from build123d import *

# Parameters (mm, degrees)
SKETCH1_W                = 100
SKETCH1_H                = 64
BOSS_EXTRUDE1_DEPTH      = 3
SKETCH2_W                = 100
SKETCH2_H                = 64
SKETCH2_W_2              = 96
SKETCH2_H_2              = 60
BOSS_EXTRUDE2_DEPTH      = 35
SKETCH6_R                = 3
SKETCH6_R_2              = 1.6
BOSS_EXTRUDE3_DEPTH      = 10
SKETCH7_R                = 1.5
CUT_EXTRUDE2_DEPTH       = 69.912988616
BOSS_EXTRUDE8_START      = -10
SKETCH10_R               = 3
SKETCH10_W               = 10
SKETCH10_H               = 10.5
SKETCH10_H_2             = 10
BOSS_EXTRUDE8_DEPTH      = 6
SKETCH11_R               = 3
CUT_EXTRUDE4_DEPTH       = 3
BOSS_EXTRUDE9_DEPTH      = 5
BOSS_EXTRUDE9_DEPTH_BACK = 37
SKETCH12_W               = 5
SKETCH12_H               = 5
SKETCH13_W               = 5.5
SKETCH13_H               = 5.5
CUT_EXTRUDE5_DEPTH       = 7
FILLET1_R                = 10


with BuildPart() as part:
    # Sketch1 → Boss-Extrude1 (new body)
    with BuildSketch(Plane(origin=(0, 0, 0), x_dir=(1, 0, 0), z_dir=(0, 1, 0))):
        Rectangle(SKETCH1_W, SKETCH1_H)
    extrude(amount=BOSS_EXTRUDE1_DEPTH)

    # Sketch2 → Boss-Extrude2 (add)
    with BuildSketch(Plane(origin=(0, 3, 0), x_dir=(1, 0, 0), z_dir=(0, 1, 0))):
        Rectangle(SKETCH2_W, SKETCH2_H)
        Rectangle(SKETCH2_W_2, SKETCH2_H_2, mode=Mode.SUBTRACT)
    extrude(amount=BOSS_EXTRUDE2_DEPTH)

    # Sketch6 → Boss-Extrude3 (add)
    # profile 1 of 4: a face of its own
    with BuildSketch(Plane(origin=(0, 3, 0), x_dir=(1, 0, 0), z_dir=(0, 1, 0))):
        with Locations(Location((-39, 25.5, 0), (0, 0, 270))):
            Circle(SKETCH6_R)
        with Locations(Location((-39, 25.5, 0), (0, 0, 270))):
            Circle(SKETCH6_R_2, mode=Mode.SUBTRACT)
    # profile 2 of 4: a face of its own
    with BuildSketch(Plane(origin=(0, 3, 0), x_dir=(1, 0, 0), z_dir=(0, 1, 0))):
        with Locations(Location((19, 25.5, 0), (0, 0, 270))):
            Circle(SKETCH6_R)
        with Locations(Location((19, 25.5, 0), (0, 0, 270))):
            Circle(SKETCH6_R_2, mode=Mode.SUBTRACT)
    # profile 3 of 4: a face of its own
    with BuildSketch(Plane(origin=(0, 3, 0), x_dir=(1, 0, 0), z_dir=(0, 1, 0))):
        with Locations(Location((-39, -23.5, 0), (0, 0, 270))):
            Circle(SKETCH6_R)
        with Locations(Location((-39, -23.5, 0), (0, 0, 270))):
            Circle(SKETCH6_R_2, mode=Mode.SUBTRACT)
    # profile 4 of 4: a face of its own
    with BuildSketch(Plane(origin=(0, 3, 0), x_dir=(1, 0, 0), z_dir=(0, 1, 0))):
        with Locations(Location((19, -23.5, 0), (0, 0, 270))):
            Circle(SKETCH6_R)
        with Locations(Location((19, -23.5, 0), (0, 0, 270))):
            Circle(SKETCH6_R_2, mode=Mode.SUBTRACT)
    extrude(amount=BOSS_EXTRUDE3_DEPTH)

    # Sketch7 → Cut-Extrude2 (cut, through all)
    with BuildSketch(Plane(origin=(0, 3, 0), x_dir=(1, 0, 0), z_dir=(0, 1, 0))):
        with Locations(Location((-39, 25.5, 0), (0, 0, 270))):
            Circle(SKETCH7_R)
        with Locations(Location((19, 25.5, 0), (0, 0, 270))):
            Circle(SKETCH7_R)
        with Locations(Location((19, -23.5, 0), (0, 0, 270))):
            Circle(SKETCH7_R)
        with Locations(Location((-39, -23.5, 0), (0, 0, 270))):
            Circle(SKETCH7_R)
    extrude(amount=-CUT_EXTRUDE2_DEPTH, mode=Mode.SUBTRACT)

    # Sketch10 → Boss-Extrude8 (add)
    # profile 1 of 6: a face of its own
    with BuildSketch(Plane(origin=(0, 13, 0), x_dir=(1, 0, 0), z_dir=(0, 1, 0)).offset(BOSS_EXTRUDE8_START)):
        with BuildLine():
            Line((-33, 25.5), (-33, 30))
            Line((-33, 30), (-48, 30))
            Line((-48, 30), (-48, 19.5))
            Line((-48, 19.5), (-39, 19.5))
            ThreePointArc((-39, 19.5), (-34.757359313, 21.257359313), (-33, 25.5))
        make_face()
        with Locations(Location((-39, 25.5, 0), (0, 0, 270))):
            Circle(SKETCH10_R, mode=Mode.SUBTRACT)
    # profile 2 of 6: a face of its own
    with BuildSketch(Plane(origin=(0, 13, 0), x_dir=(1, 0, 0), z_dir=(0, 1, 0)).offset(BOSS_EXTRUDE8_START)):
        with BuildLine():
            Line((25, 25.5), (25, 30))
            Line((25, 30), (13, 30))
            Line((13, 30), (13, 25.5))
            ThreePointArc((13, 25.5), (19, 19.5), (25, 25.5))
        make_face()
        with Locations(Location((19, 25.5, 0), (0, 0, 270))):
            Circle(SKETCH10_R, mode=Mode.SUBTRACT)
    # profile 3 of 6: a face of its own
    with BuildSketch(Plane(origin=(0, 13, 0), x_dir=(1, 0, 0), z_dir=(0, 1, 0)).offset(BOSS_EXTRUDE8_START)):
        with BuildLine():
            Line((25, -23.5), (25, -30))
            Line((25, -30), (13, -30))
            Line((13, -30), (13, -23.5))
            ThreePointArc((13, -23.5), (19, -17.5), (25, -23.5))
        make_face()
        with Locations(Location((19, -23.5, 0), (0, 0, 270))):
            Circle(SKETCH10_R, mode=Mode.SUBTRACT)
    # profile 4 of 6: a face of its own
    with BuildSketch(Plane(origin=(0, 13, 0), x_dir=(1, 0, 0), z_dir=(0, 1, 0)).offset(BOSS_EXTRUDE8_START)):
        with BuildLine():
            Line((-33, -23.5), (-33, -30))
            Line((-33, -30), (-48, -30))
            Line((-48, -30), (-48, -17.5))
            Line((-48, -17.5), (-39, -17.5))
            ThreePointArc((-39, -17.5), (-34.757359313, -19.257359313), (-33, -23.5))
        make_face()
        with Locations(Location((-39, -23.5, 0), (0, 0, 270))):
            Circle(SKETCH10_R, mode=Mode.SUBTRACT)
    # profile 5 of 6: a face of its own
    with BuildSketch(Plane(origin=(0, 13, 0), x_dir=(1, 0, 0), z_dir=(0, 1, 0)).offset(BOSS_EXTRUDE8_START)):
        with Locations((43, 24.75)):
            Rectangle(SKETCH10_W, SKETCH10_H)
    # profile 6 of 6: a face of its own
    with BuildSketch(Plane(origin=(0, 13, 0), x_dir=(1, 0, 0), z_dir=(0, 1, 0)).offset(BOSS_EXTRUDE8_START)):
        with Locations((43, -25)):
            Rectangle(SKETCH10_W, SKETCH10_H_2)
    extrude(amount=BOSS_EXTRUDE8_DEPTH)

    # Sketch11 → Cut-Extrude4 (cut)
    with BuildSketch(Plane.XZ):
        with Locations(Location((-39, 23.5, 0), (0, 0, 90))):
            Circle(SKETCH11_R)
        with Locations(Location((19, 23.5, 0), (0, 0, 90))):
            Circle(SKETCH11_R)
        with Locations(Location((19, -25.5, 0), (0, 0, 90))):
            Circle(SKETCH11_R)
        with Locations(Location((-39, -25.5, 0), (0, 0, 90))):
            Circle(SKETCH11_R)
        with BuildLine():
            Line((-46, -10), (-46, 10))
            ThreePointArc((-46, 10), (-41, 15), (-36, 10))
            Line((-36, 10), (-36, -10))
            ThreePointArc((-36, -10), (-41, -15), (-46, -10))
        make_face()
    extrude(amount=-CUT_EXTRUDE4_DEPTH, mode=Mode.SUBTRACT)

    # Sketch12 → Boss-Extrude9 (add, two sides: drawn at the far end of the back side and taken through both)
    with BuildSketch(Plane(origin=(0, 38, 0), x_dir=(1, 0, 0), z_dir=(0, 1, 0)).offset(-BOSS_EXTRUDE9_DEPTH_BACK)):
        with Locations((-45.5, 27.5)):
            Rectangle(SKETCH12_W, SKETCH12_H)
        with Locations((45.5, 27.5)):
            Rectangle(SKETCH12_W, SKETCH12_H)
        with Locations((45.5, -27.5)):
            Rectangle(SKETCH12_W, SKETCH12_H)
        with Locations((-45.5, -27.5)):
            Rectangle(SKETCH12_W, SKETCH12_H)
    extrude(amount=BOSS_EXTRUDE9_DEPTH + BOSS_EXTRUDE9_DEPTH_BACK)

    # Sketch13 → Cut-Extrude5 (cut)
    with BuildSketch(Plane.XZ):
        with Locations((-45.25, 27.25)):
            Rectangle(SKETCH13_W, SKETCH13_H)
        with Locations((-45.25, -27.25)):
            Rectangle(SKETCH13_W, SKETCH13_H)
        with Locations((45.25, -27.25)):
            Rectangle(SKETCH13_W, SKETCH13_H)
        with Locations((45.25, 27.25)):
            Rectangle(SKETCH13_W, SKETCH13_H)
    extrude(amount=-CUT_EXTRUDE5_DEPTH, mode=Mode.SUBTRACT)

    # Fillet1
    fillet1_edges = [part.edges().sort_by_distance(p)[0] for p in [
        (38, 6, 20),
        (38, 6, -19.5),
    ]]
    fillet(fillet1_edges, radius=FILLET1_R - 0.0001)  # a hair under: the kernel refuses the full size


solid = part.part
Input: part model. Units: mm. Frame: model coordinates. A direction names the side the tool comes from. Coordinates: 2 decimals unless noted, no trailing zeros. Order: outer loops, then holes, each group sorted by start corner. A loop starts at its lowest first (then second) coordinate and runs counter-clockwise, first axis right, second up.
1. Cut plane C-C, the plane x = -31. Return loops of the section in (y, z).
Checked values:
outline: (0, -32) - (38, -32) - (38, -30) - (3, -30) - (3, 30) - (38, 30) - (38, 32) - (0, 32) - close
2. Cut plane D-D, the plane x = 19. Count the separate pieces of the cut face and the enclosed holes in it, plus the area to 3 significant figures.
Checked values:
separate pieces: 3
enclosed holes: 0
area: 418 mm2
3. Access query for faces 4 (the flat face through (-46, 40, -30)), 5 (the cylindrical face through (40.85, 6.04, 23.01)), 6 (the flat face through (-42.5, 3, 27)). Directions: +Z, -Z, +X, -X, +Y, -Y. A direction counts if a zero-diameter tool reaches every point of the face in a straight line with its end or side. Return the directions, or none.
Checked values:
face 4: -Z, +X, -X, +Y
face 5: +Y
face 6: -Y
4. Contact query for flat-ended pins moving along their axis: P1, Ø3, axis at x = -39.5, z = -26.5, coming from the -Y side; P2, Ø8, axis at x = -39, z = 23.5, coming from the +Y side; P3, Ø5.5, axis at y = 41.5, z = -27, coming from the -X side. Output: stop coordinate, or through.
Checked values:
P1: stops at y = 3
P2: stops at y = 13
P3: stops at x = -48
5. Ray query, line 1 along X through (y, z) = (1, -25.5); line 2 along X through (y, z) = (8, -5); line 3 along Z through (x, y) = (19, 1). Return the intervals inside material, ascending.
Checked values:
line 1: x = -50 to -48, -42.5 to -42, -36 to 16, 22 to 42.5, 48 to 50
line 2: x = -50 to -48, 48 to 50
line 3: z = -32 to -28.5, -22.5 to 20.5, 26.5 to 32
6. Cut plane A-A, the plane y = 17. Return loops of the section in (x, z).
Checked values:
outline: (-50, -32) - (50, -32) - (50, 32) - (-50, 32) - close; hole (-48, -25) - (-43, -25) - (-43, -30) - (43, -30) - (43, -25) - (48, -25) - (48, 25) - (43, 25) - (43, 30) - (-43, 30) - (-43, 25) - (-48, 25) - close
7. Draft query along Z for faces 1 (the flat face through (-1, 19, -32)), 2 (the flat face through (18, 13, -24)), 3 (the flat face through (-48, 40, -27)). Return one class per face: +Z half, -Z half, draft (parallel to the pull), parting line (faces both ways), or undercut.
Checked values:
face 1: -Z half
face 2: undercut
face 3: draft
8. Cut plane B-B, the plane z = -4.5. Return loops of the section in (x, y), plus the area to 3 significant figures.
Checked values:
outline: (-50, 0) - (-46, 0) - (-46, 3) - (-48, 3) - (-48, 38) - (-50, 38) - close; (-36, 0) - (50, 0) - (50, 38) - (48, 38) - (48, 3) - (-36, 3) - close
area: 410 mm2
